Work out the finished part from the listing and answer in its coordinate system (mm). A direction names the side the tool comes from. Coordinates: 2 decimals unless noted, no trailing zeros. Write each loop counter-clockwise with the first axis right and the second up, starting at its lowest first coordinate (ties: lowest second). Pieces come first, ordered by that corner, then holes. Notation, with made-up numbers: M -18.5,-22 L 31.5,-22 A16 cw 31.5,-14 Z; hole C 4,81.25 d1. An arc over 180 degrees is marked long. Use CSV: the item, a comma, the result in double quotes.
from build123d import *

# Parameters (mm, degrees)
F1_DEPTH = 20
F2_R     = 5
F3_T     = -4


with BuildPart() as f1:
    # F0 (on Top) → F1 (new body)
    with BuildSketch(Plane.XY):
        with BuildLine():
            ThreePointArc((30, 0), (51.2132034356, 8.7867965644), (60, 30))
            ThreePointArc((60, 30), (37.6347989784, 59.0122361179), (3.8860103627, 44.7668393782))
            ThreePointArc((3.8860103627, 44.7668393782), (0.4502981981, 35.1783321081), (0.4207995235, 24.9929151026))
            ThreePointArc((0.4207995235, 24.9929151026), (8.9863784152, 21.1887860474), (12.5, 12.5))
            ThreePointArc((12.5, 12.5), (12.1402716069, 9.5227856456), (11.0817911501, 6.716929457))
            ThreePointArc((11.0817911501, 6.716929457), (19.9623736942, 1.7290598291), (30, 0))
        make_face()
        with BuildLine():
            ThreePointArc((0.4207995235, 24.9929151026), (0.4502981981, 35.1783321081), (3.8860103627, 44.7668393782))
            Line((3.8860103627, 44.7668393782), (-10.8808290155, 18.6528497409))
            ThreePointArc((-10.8808290155, 18.6528497409), (-6.1157306547, 23.4017355755), (0.4207995235, 24.9929151026))
        make_face()
        with BuildLine():
            Line((0, 0), (30, 0))
            ThreePointArc((30, 0), (19.9623736942, 1.7290598291), (11.0817911501, 6.716929457))
            ThreePointArc((11.0817911501, 6.716929457), (6.4792599196, 1.8103231623), (0, 0))
        make_face()
        with BuildLine():
            ThreePointArc((11.0817911501, 6.716929457), (4.086632973, 14.8838692343), (0.4207995235, 24.9929151026))
            ThreePointArc((0.4207995235, 24.9929151026), (-6.1157306547, 23.4017355755), (-10.8808290155, 18.6528497409))
            ThreePointArc((-10.8808290155, 18.6528497409), (-10.7972362612, 6.2016121809), (0, 0))
            ThreePointArc((0, 0), (6.4792599196, 1.8103231623), (11.0817911501, 6.716929457))
        make_face()
        with BuildLine():
            ThreePointArc((12.5, 12.5), (8.9863784152, 21.1887860474), (0.4207995235, 24.9929151026))
            ThreePointArc((0.4207995235, 24.9929151026), (4.086632973, 14.8838692343), (11.0817911501, 6.716929457))
            ThreePointArc((11.0817911501, 6.716929457), (12.1402716069, 9.5227856456), (12.5, 12.5))
        make_face()
    extrude(amount=F1_DEPTH)

    # F2
    f2_edges = [f1.edges().sort_by_distance(p)[0] for p in [
        (55.913367, 45.116131, 20),
        (-3.497409, 31.709845, 20),
        (-10.797236, 6.201612, 20),
        (15, 0, 20),
    ]]
    fillet(f2_edges, radius=F2_R)

    # F3
    f3_openings = [f1.faces().sort_by_distance(p)[0] for p in [
        (25.443673, 27.342143, 0),
    ]]
    offset(amount=F3_T, openings=f3_openings)


solid = f1.part
Item 1: The part is cut by section A-A (z = 11.75). Write down the section's boundary in (x, y).
Answer:
outline,"M -10.88,18.65 A12.5 ccw 0,0 L 30,0 A30 ccw long 3.89,44.77 Z; hole M -7.4,16.68 A8.5 ccw 0,4 L 30,4 A26 ccw long 7.37,42.8 Z"
Item 2: A tool of negligible diameter and unlimited length cuts with its end or side. For faces 5 (the face through (-10.89, 6.36, 7.4)), 6 (the face through (-7.4, 8.32, 7.4)), from which of +Z, -Z, +X, -X, +Y, -Y can it reach the whole face along a straight path? Write none if from no direction.
Answer:
face 5,"+Z, -Z, -X"
face 6,"-Z"
Item 3: Consider probe 1 along Z at (x, y) = (38.5, 24.5); probe 2 along X at (y, z) = (7, 1); probe 3 along X at (y, z) = (37.5, 3.75). Determine where each line is inside the solid, lowest interval first.
Answer:
probe 1,"z = 16 to 20"
probe 2,"x = -11.22 to -6.48, 42.12 to 49.26"
probe 3,"x = -0.22 to 4.37, 54.89 to 59.05"
Item 4: For a pull along Y with two mould halves and no side action, classify faces 1 (the face through (15, 4, 7)), 2 (the face through (5, 39, 0)), 3 (the face through (15, 0, 7)), 4 (the face through (23, 30, 16)) as released by +Y, released by -Y, zero draft, split by the parting line, or undercut.
Answer:
face 1,"undercut"
face 2,"zero draft"
face 3,"released by -Y"
face 4,"undercut"
Item 5: Given pin 1 (12 mm diameter, centred on x = -1, z = 3.5, fed in from +Y); pin 2 (2 mm diameter, centred on x = 52.5, y = 27.5, fed in from -Z); pin 3 (12 mm diameter, centred on x = 8.5, z = 7.5, fed in from +Y), each flat-ended and moving along its own axis, determine where each tip first touches the part or whether it passes through.
Answer:
pin 1,"stops at y = 46.58"
pin 2,"stops at z = 16"
pin 3,"stops at y = 55.69"
